from build123d import *

# Parameters (mm, degrees)
F0_W      = 508
F0_H      = 254
F0_R      = 62.653986
F1_DEPTH  = 25.4
F1_FACE_W = 508
F1_FACE_H = 254
F1_FACE_R = 62.653986
F2_DEPTH  = 25.4
F3_W      = 40.465146
F3_H      = 254
F4_DEPTH  = 25.4


with BuildPart() as f1:
    # F0 (on Top) → F1 (new body)
    with BuildSketch(Plane.XY):
        with Locations((108.643128, 113.547525)):
            Rectangle(F0_W, F0_H)
        with Locations((108.643128, 113.547525)):
            Circle(F0_R, mode=Mode.SUBTRACT)
    extrude(amount=F1_DEPTH)

    # F1_face (on face) → F2 (join)
    with BuildSketch(Plane(origin=(108.643128, 113.547525, 25.4), x_dir=(1, 0, 0), z_dir=(0, 0, 1))):
        Rectangle(F1_FACE_W, F1_FACE_H)
        Circle(F1_FACE_R, mode=Mode.SUBTRACT)
    extrude(amount=F2_DEPTH)

    # F3 (on face) → F4 (cut)
    with BuildSketch(Plane.XY.offset(50.8)):
        with Locations((-56.300491, 113.547525)):
            Rectangle(F3_W, F3_H)
    extrude(amount=-F4_DEPTH, mode=Mode.SUBTRACT)


solid = f1.part
Verification items for the finished model (mm, model axes). A direction names the side the tool comes from. Give positions to 0.01 mm unless a question says otherwise; leave off trailing zeros. Loops run counter-clockwise (first coordinate to the right, second up) from the corner with the lowest first, then second, coordinate; pieces in that order, holes last.
1) Set-up check for faces 1 (the flat face through (205, 115, 50.8)), 2 (the flat face through (-57, 115, 25.4)): record each of +Z, -Z, +X, -X, +Y, -Y from which the full face is reachable in a straight line by a thin tool's end or side.
2) Thickness scan on line 1 along X through (y, z) = (187, 48.5); line 2 along X through (y, z) = (68, 38); line 3 along X through (y, z) = (125.5, 47). Record the ranges inside material, lowest first.
3) Draft check along X on faces 3 (the flat face through (362.643, 112, 25)), 4 (the flat face through (49, 144, 0)), 5 (the cylindrical face through (95.061, 52.383, 25.044)), 6 (the flat face through (-145.357, 112, 25)). Enter one of: pulls with the +X half, pulls with the -X half, needs draft (parallel to the pull), parting line crosses it, or undercut.
4) Depth check by flat-ended pin: pin 1 Ø20 at (x, y) = (-61.5, 119) entering from +Z. Enter the tip coordinate at first touch or a pass-through.
5) Sectioned sample at C-C, the plane x = 52.5. Enter the section's corners in (y, z).
6) Sectioned sample at A-A, the plane y = 7.5. Enter the section's corners in (x, z), then the cut area to 3 significant figures.
7) Sectioned sample at B-B, the plane z = 44. Enter the section's corners in (x, y), then the cut area to 3 significant figures.
8) Sectioned sample at D-D, the plane y = 98.5. Enter the section's corners in (x, z), then the cut area to 3 significant figures.
Answers:
1. face 1: +Z, +X, -X, +Y, -Y
1. face 2: +Z, +Y, -Y
2. line 1: x = -145.36 to -76.53, -36.07 to 362.64
2. line 2: x = -145.36 to -76.53, -36.07 to 65.62, 151.67 to 362.64
2. line 3: x = -145.36 to -76.53, -36.07 to 47.14, 170.15 to 362.64
3. face 3: pulls with the +X half
3. face 4: needs draft
3. face 5: undercut
3. face 6: pulls with the -X half
4. pin 1: stops at z = 25.4
5. outline: (-13.45, 0) - (85.74, 0) - (85.74, 50.8) - (-13.45, 50.8) - close; (141.36, 0) - (240.55, 0) - (240.55, 50.8) - (141.36, 50.8) - close
6. outline: (-145.36, 0) - (362.64, 0) - (362.64, 50.8) - (-36.07, 50.8) - (-36.07, 25.4) - (-76.53, 25.4) - (-76.53, 50.8) - (-145.36, 50.8) - close
6. area: 24,800 mm2
7. outline: (-145.36, -13.45) - (-76.53, -13.45) - (-76.53, 240.55) - (-145.36, 240.55) - close; (-36.07, -13.45) - (362.64, -13.45) - (362.64, 240.55) - (-36.07, 240.55) - close; hole circle Ø125.31 at (108.64, 113.55)
7. area: 106,000 mm2
8. outline: (-145.36, 0) - (47.82, 0) - (47.82, 50.8) - (-36.07, 50.8) - (-36.07, 25.4) - (-76.53, 25.4) - (-76.53, 50.8) - (-145.36, 50.8) - close; (169.46, 0) - (362.64, 0) - (362.64, 50.8) - (169.46, 50.8) - close
8. area: 18,600 mm2
